Part model, mm, in its own coordinate system. A direction names the side the tool comes from. Coordinates: 2 decimals unless noted, no trailing zeros. Write each loop counter-clockwise with the first axis right and the second up, starting at its lowest first coordinate (ties: lowest second). Pieces come first, ordered by that corner, then holes. Notation, with made-up numbers: (24, 28.25) - (81, 28.25) arc R33 ccw to (81, 60.25) - close; hole circle Ø5 at (76.25, 88). An arc over 180 degrees is marked (long way). Write each question's results on one line, items separated by ' | '.
from build123d import *

# Parameters (mm, degrees)
F0_W     = 76.2
F0_H     = 76.2
F1_DEPTH = 6.35


with BuildPart() as f1:
    # F0 (on Top) → F1 (new body)
    with BuildSketch(Plane.XY):
        Rectangle(F0_W, F0_H)
        with BuildLine():
            ThreePointArc((-7.921258, -27.766384), (-13.068427, -28.129462), (-13.431505, -22.982294))
            Line((-13.431505, -22.982294), (19.872915, 15.377263))
            ThreePointArc((19.872915, 15.377263), (25.020084, 15.740341), (25.383162, 10.593172))
            Line((25.383162, 10.593172), (-7.921258, -27.766384))
        make_face(mode=Mode.SUBTRACT)
        with BuildLine():
            ThreePointArc((-21.596966, -15.714419), (-26.744134, -16.077497), (-27.107213, -10.930329))
            Line((-27.107213, -10.930329), (6.197208, 27.429228))
            ThreePointArc((6.197208, 27.429228), (11.344377, 27.792306), (11.707455, 22.645137))
            Line((11.707455, 22.645137), (-21.596966, -15.714419))
        make_face(mode=Mode.SUBTRACT)
    extrude(amount=F1_DEPTH)


solid = f1.part
(1) Wall check: line 1 (X direction, y = -0.5, z = 3); line 2 (X direction, y = 4, z = 1); line 3 (Y direction, x = -5, z = 1.25). Give the ranges that are in metal, low to high. Write a range as from..to.
Return value:
line 1: x = -38.1..-18.05, -8.39..6.09, 15.75..38.1 | line 2: x = -38.1..-14.14, -4.48..9.99, 19.66..38.1 | line 3: y = -38.1..-24.4, -13.27..3.4, 14.53..38.1
(2) Saw through at B-B on y = -25. Write the cut outline in (x, z), then the cut area to 3 significant figures.
Return value:
outline: (-38.1, 0) - (-14.31, 0) - (-14.31, 6.35) - (-38.1, 6.35) - close; (-5.52, 0) - (38.1, 0) - (38.1, 6.35) - (-5.52, 6.35) - close | area: 428 mm^2
(3) Two-plate mould, pull along Y, no slides. Class faces 3 (the flat face through (-1, -38.1, 3)), 4 (the flat face through (-38.1, -1, 3)), 5 (the cylindrical face through (24.96, 15.79, 3.13)): released by +Y, released by -Y, zero draft, split by the parting line, or undercut.
Return value:
face 3: released by -Y | face 4: zero draft | face 5: undercut
(4) Saw through at D-D on x = 16. Write the cut outline in (y, z).
Return value:
outline: (-38.1, 0) - (-0.21, 0) - (-0.21, 6.35) - (-38.1, 6.35) - close; (10.92, 0) - (38.1, 0) - (38.1, 6.35) - (10.92, 6.35) - close
(5) 3-axis set-ups, long thin cutter, end or side, ignore diameter. For faces 1 (the flat face through (-4.712, 3.734, 3.131)), 2 (the flat face through (-1, 38.1, 3)): which of +Z, -Z, +X, -X, +Y, -Y reach the whole face in a straight line?
Return value:
face 1: +Z, -Z | face 2: +Z, -Z, +X, -X, +Y
(6) Saw through at C-C on x = 3. Write the cut outline in (y, z), then the cut area to 3 significant figures.
Return value:
outline: (-38.1, 0) - (-15.19, 0) - (-15.19, 6.35) - (-38.1, 6.35) - close; (-4.06, 0) - (12.62, 0) - (12.62, 6.35) - (-4.06, 6.35) - close; (23.75, 0) - (38.1, 0) - (38.1, 6.35) - (23.75, 6.35) - close | area: 343 mm^2
(7) Flat gauge pin, fed straight in: P1, Ø12, axis at x = -27.5, y = 5.5, coming from the -Z side. Where does the tip first touch, or does it go through?
Return value:
P1: stops at z = 0
(8) Saw through at A-A on z = 1.5. Write the cut outline in (x, y), then the cut area to 3 significant figures.
Return value:
outline: (-38.1, -38.1) - (38.1, -38.1) - (38.1, 38.1) - (-38.1, 38.1) - close; hole (-27.11, -10.93) arc R3.65 ccw to (-21.6, -15.71) - (11.71, 22.65) arc R3.65 ccw to (6.2, 27.43) - close; hole (-13.43, -22.98) arc R3.65 ccw to (-7.92, -27.77) - (25.38, 10.59) arc R3.65 ccw to (19.87, 15.38) - close | area: 4,980 mm^2
